from build123d import *

# Parameters (mm, degrees)
F0_R     = 6
F1_DEPTH = 15
F5_D     = 6.5
F5_DEPTH = 15
F5_TIP   = 1.9527970118
F6_SIZE  = 1


with BuildPart() as f1:
    # F0 (on Top) → F1 (new body)
    with BuildSketch(Plane.XY):
        Circle(F0_R)
    extrude(amount=F1_DEPTH)

    # F2 (on Top) → F3 (revolve)
    with BuildSketch(Plane.XY):
        with BuildLine():
            Line((-8.5, 0), (8.5, 0))
            ThreePointArc((8.5, 0), (0, 8.5), (-8.5, 0))
        make_face()
    revolve(axis=Axis((0, 0, 0), (1, 0, 0)))

    # F5
    with Locations(Plane.XY.offset(15)):
        with Locations((0, 0)):
            Hole(F5_D / 2, depth=F5_DEPTH)
            with Locations((0, 0, -(F5_DEPTH + F5_TIP / 2))):  # 118° drill point
                Cone(0, F5_D / 2, F5_TIP, mode=Mode.SUBTRACT)

    # F6
    f6_edges = [f1.edges().sort_by_distance(p)[0] for p in [
        (-6, 0, 15),
    ]]
    chamfer(f6_edges, length=F6_SIZE)


solid = f1.part
The listing builds one solid part. Answer for the finished solid, in the listing's coordinates (mm). Coordinates: 2 decimals unless noted, no trailing zeros. Order: outer loops, then holes, each group sorted by start corner. A loop starts at its lowest first (then second) coordinate and runs counter-clockwise, first axis right, second up. Notation, with made-up numbers: (36, 82.5) -> (55, 82.5) arc R28 ccw to (55, 114.5) -> close; hole circle Ø8 at (63, 77.25). An arc over 180 degrees is marked (long way). Answer in a Markdown table with one row per item. Add a question column.
Item 1: Find section B-B (z = -2.25). Write down the section's boundary in (x, y), then the cut area to 3 significant figures.
Item 2: Find section A-A (z = -5.25). Write down the section's boundary in (x, y).
Item 3: Each of these flat-tipped pins is pushed along its axis until it touches: P1, Ø3, axis at y = -4.5, z = 9, coming from the -X side; P2, Ø3, axis at x = 2.5, z = 10, coming from the -Y side; P3, Ø6, axis at x = -4, z = 1, coming from the -Y side. Where does it stop, or does it pass through?
Item 4: Find the intervals of material crossed by L1, parallel to Y at x = 0, z = 7.25; L2, parallel to Y at x = 0, z = 5.5, in increasing order. Write a range as from..to.
Item 5: Determine the mould class of faces 1 (the face through (-6, 0, 10)), 2 (the face through (2.579, -1.978, 7.395)), 3 (the face through (1, -3.3, 15)) for opening direction X: +X half, -X half, draft (parallel to the pull), parting line (faces both ways), or undercut.
Result set:
| question | item | result |
|---|---|---|
| 1 | outline | circle Ø16.39 at (0, 0) |
| 1 | area | 211 mm² |
| 2 | outline | circle Ø13.37 at (0, 0) |
| 3 | P1 | stops at x = -5.2 |
| 3 | P2 | stops at y = -5.92 |
| 3 | P3 | stops at y = -8.43 |
| 4 | L1 | y = -6..-3.25, 3.25..6 |
| 4 | L2 | y = -6.48..-3.25, 3.25..6.48 |
| 5 | face 1 | parting line |
| 5 | face 2 | undercut |
| 5 | face 3 | draft |
